For this review, take the finished solid that the model builds, in its own axes (mm). Round coordinates to 2 decimals unless told otherwise and drop trailing zeros. Write each loop counter-clockwise with the first axis right and the second up, starting at its lowest first coordinate (ties: lowest second). Pieces come first, ordered by that corner, then holes. Notation, with made-up numbers: (79.25, -31.5) -> (84.25, -31.5) arc R35 cw to (84.25, 6.5) -> close; hole circle Ø4 at (-1, 51.25). An arc over 180 degrees is marked (long way). Answer in a Markdown table with one row per item.
from build123d import *

# Parameters (mm, degrees)
SKETCH_1_W          = 300
SKETCH_1_H          = 100
EXTRUDE_1_DEPTH     = 1.8
SKETCH_2_W          = 100
SKETCH_2_H          = 50
CUT_EXTRUDE_1_DEPTH = 2.8
SKETCH_3_R          = 2
SKETCH_3_R_2        = 10
CUT_EXTRUDE_2_DEPTH = 2.8


with BuildPart() as part:
    # 草图1 → 凸台-拉伸1 (new body)
    with BuildSketch(Plane(origin=(0, 0, 0), x_dir=(1, 0, 0), z_dir=(0, 1, 0))):
        with Locations((150, 50)):
            Rectangle(SKETCH_1_W, SKETCH_1_H)
    extrude(amount=EXTRUDE_1_DEPTH)

    # 草图2 → 切除-拉伸1 (cut, through all)
    with BuildSketch(Plane(origin=(0, 1.8, 0), x_dir=(1, 0, 0), z_dir=(0, 1, 0))):
        with Locations((50, 75)):
            Rectangle(SKETCH_2_W, SKETCH_2_H)
    extrude(amount=-CUT_EXTRUDE_1_DEPTH, mode=Mode.SUBTRACT)

    # 草图3 → 切除-拉伸2 (cut, through all)
    with BuildSketch(Plane(origin=(0, 1.8, 0), x_dir=(1, 0, 0), z_dir=(0, 1, 0))):
        with Locations((95, 35)):
            Circle(SKETCH_3_R)
        with Locations((75, 35)):
            Circle(SKETCH_3_R)
        with Locations((75, 15)):
            Circle(SKETCH_3_R)
        with Locations((95, 15)):
            Circle(SKETCH_3_R)
        with Locations((85, 25)):
            Circle(SKETCH_3_R_2)
    extrude(amount=-CUT_EXTRUDE_2_DEPTH, mode=Mode.SUBTRACT)


solid = part.part
1) Consider section B-B on y = 0.8. State the section outline as (x, z) points.
Solved:
| item | result |
|---|---|
| outline | (0, -50) -> (100, -50) -> (100, -100) -> (300, -100) -> (300, 0) -> (0, 0) -> close; hole circle Ø4 at (75, -35); hole circle Ø4 at (75, -15); hole circle Ø20 at (85, -25); hole circle Ø4 at (95, -35); hole circle Ø4 at (95, -15) |
2) Clearance check with a flat-ended pin moving along its axis: pin 1 Ø0.9 at (x, y) = (72, 1) entering from -Z. State where the tip first meets the part, or that it passes through.
Solved:
| item | result |
|---|---|
| pin 1 | z = -50 |
3) Consider section A-A on z = -25. State the section outline as (x, y) points.
Solved:
| item | result |
|---|---|
| outline | (0, 0) -> (75, 0) -> (75, 1.8) -> (0, 1.8) -> close; (95, 0) -> (300, 0) -> (300, 1.8) -> (95, 1.8) -> close |
4) Mouldability with a two-part tool opening along X and no side actions: class faces 1 (the cylindrical face through (75, 1, -25)), 2 (the flat face through (181, 1.8, -51)) as pulls with the +X half, pulls with the -X half, needs draft (parallel to the pull), parting line crosses it, or undercut.
Solved:
| item | result |
|---|---|
| face 1 | undercut |
| face 2 | needs draft |
5) For line 1 (X direction, y = 1.7, z = -28.5); line 2 (Z direction, x = 93.5, y = 0.9); line 3 (Z direction, x = 85, y = 1), list the stretches that pass through material, from the lowest coordinate up. Write a range as [from, to].
Solved:
| item | result |
|---|---|
| line 1 | [0, 75.63], [94.37, 300] |
| line 2 | [-50, -36.32], [-33.68, -30.27], [-19.73, -16.32], [-13.68, 0] |
| line 3 | [-50, -35], [-15, 0] |
6) Consider section D-D on x = 19. State the section outline as (y, z) points.
Solved:
| item | result |
|---|---|
| outline | (0, -50) -> (1.8, -50) -> (1.8, 0) -> (0, 0) -> close |
7) Consider section C-C on x = 84. State the section outline as (y, z) points.
Solved:
| item | result |
|---|---|
| outline | (0, -50) -> (1.8, -50) -> (1.8, -34.95) -> (0, -34.95) -> close; (0, -15.05) -> (1.8, -15.05) -> (1.8, 0) -> (0, 0) -> close |
